Design review of the part built by this model. Coordinates are the model's own, in mm. Face numbers are marked on the shaded views. A direction names the side the tool comes from. Round coordinates to 2 decimals unless told otherwise and drop trailing zeros. Write each loop counter-clockwise with the first axis right and the second up, starting at its lowest first coordinate (ties: lowest second). Pieces come first, ordered by that corner, then holes. Notation, with made-up numbers: M 6.5,-25.5 L 12.5,-25.5 A34 ccw 12.5,4.5 Z; hole C 61.25,44 d9. An arc over 180 degrees is marked long. One line per question, with ' | ' between items. Start each with the question number.
Item 1: Add section B-B, the plane y = 10. State the section outline as (x, z) points.
Item 2: Insertion check: pin 1 Ø5 at (x, z) = (3, -9) entering from -Y; pin 2 Ø5 at (x, y) = (18, 0) entering from +Z; pin 3 Ø5 at (x, y) = (-26.5, 4) entering from +Z; pin 4 Ø1 at (x, y) = (-5, 11) entering from +Z. Each pin has a flat end and moves straight along its axis. Give the tip position at first contact, or say it passes through.
Item 3: For L1, parallel to Y at x = 0, z = -10; L2, parallel to Y at x = -18, z = -39.25; L3, parallel to Y at x = 30, z = -30, list the stretches that pass through material, from the lowest coordinate up.
Item 4: Add section C-C, the plane x = -18. Give the number of separate pieces and of enclosed holes in the cut face, and give its area (3 significant figures).
Item 5: Add section A-A, the plane x = 0. State the section outline as (y, z) points.
Item 6: Draft analysis for pull direction Y (two halves, no side actions). For the marked faces 4, 5 and 6, state which applies: released by +Y, released by -Y, zero draft, split by the parting line, or undercut.
Item 7: Machinability: for the marked faces 1, 2 and 3, which of the approach directions +Z, -Z, +X, -X, +Y, -Y give a long, thin tool a straight path to every point of the face, cutting with its end or side? Answer none if there is none.
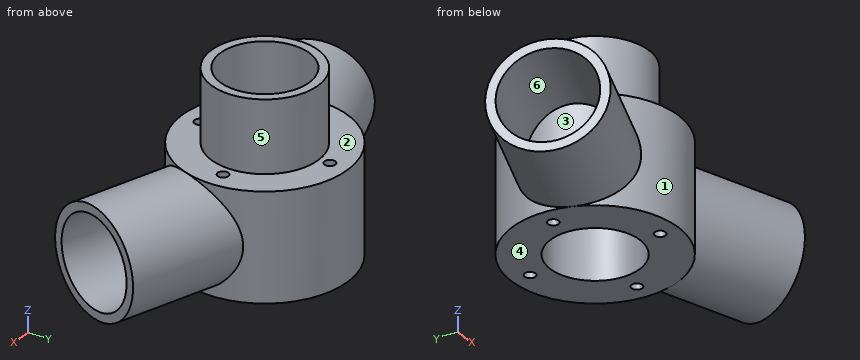
```python
from build123d import *

# Parameters (mm, degrees)
CROQUIS1_R              = 15
CROQUIS1_R_2            = 12.5
SALIENTE_EXTRUIR1_DEPTH = 20
CROQUIS8_R              = 23.25
CROQUIS8_R_2            = 1.5
SALIENTE_EXTRUIR2_DEPTH = 30
SALIENTE_EXTRUIR4_REACH = 81.8
CROQUIS6_R              = 15
CROQUIS6_R_2            = 12.5
SALIENTE_EXTRUIR5_REACH = 108.924
CROQUIS7_R              = 15
CROQUIS7_R_2            = 12.5
CROQUIS9_R              = 12.5
CORTAR_EXTRUIR1_DEPTH   = 31.000000103


with BuildPart() as part:
    # Croquis1 → Saliente-Extruir1 (new body)
    with BuildSketch(Plane.XY):
        Circle(CROQUIS1_R)
        Circle(CROQUIS1_R_2, mode=Mode.SUBTRACT)
    extrude(amount=-SALIENTE_EXTRUIR1_DEPTH)

    # Croquis8 → Saliente-Extruir2 (add)
    with BuildSketch(Plane(origin=(0, 0, -20), x_dir=(-1, 0, 0), z_dir=(0, 0, -1))):
        Circle(CROQUIS8_R)
        with Locations((0, 18)):
            Circle(CROQUIS8_R_2, mode=Mode.SUBTRACT)
        with Locations((18, 0)):
            Circle(CROQUIS8_R_2, mode=Mode.SUBTRACT)
        with Locations((0, -18)):
            Circle(CROQUIS8_R_2, mode=Mode.SUBTRACT)
        with Locations((-18, 0)):
            Circle(CROQUIS8_R_2, mode=Mode.SUBTRACT)
    extrude(amount=SALIENTE_EXTRUIR2_DEPTH)

    # Croquis6 → Saliente-Extruir4 (add, up to next)
    with BuildSketch(Plane(origin=(46.984631039, -17.101007166, -35), x_dir=(0, 0, -1), z_dir=(0.939692621, -0.342020143, 0)), mode=Mode.PRIVATE) as saliente_extruir4_sk1:
        Circle(CROQUIS6_R)
        Circle(CROQUIS6_R_2, mode=Mode.SUBTRACT)
    saliente_extruir4_tool1 = extrude(saliente_extruir4_sk1.sketch, amount=-SALIENTE_EXTRUIR4_REACH, mode=Mode.PRIVATE) - part.part
    add(saliente_extruir4_tool1.solids().sort_by_distance((46.984631, -17.101007, -20.424264))[0])

    # Croquis7 → Saliente-Extruir5 (add, up to next)
    with BuildSketch(Plane(origin=(-46.984631039, -17.101007166, -35), x_dir=(0, 0, 1), z_dir=(-0.939692621, -0.342020143, 0)), mode=Mode.PRIVATE) as saliente_extruir5_sk1:
        Circle(CROQUIS7_R)
        Circle(CROQUIS7_R_2, mode=Mode.SUBTRACT)
    saliente_extruir5_tool1 = extrude(saliente_extruir5_sk1.sketch, amount=-SALIENTE_EXTRUIR5_REACH, mode=Mode.PRIVATE) - part.part
    add(saliente_extruir5_tool1.solids().sort_by_distance((-46.984631, -17.101007, -49.575736))[0])

    # Croquis9 → Cortar-Extruir1 (cut, through all)
    with BuildSketch(Plane.XY.offset(-20)):
        Circle(CROQUIS9_R)
    extrude(amount=-CORTAR_EXTRUIR1_DEPTH, mode=Mode.SUBTRACT)


solid = part.part
```
Computed values:
1) outline: M -20.99,-50 L -7.5,-50 L -7.5,0 L -11.18,0 L -11.18,-20 L -20.99,-20 Z; M 7.5,-50 L 20.99,-50 L 20.99,-20 L 11.18,-20 L 11.18,0 L 7.5,0 Z
2) pin 1: stops at y = -14.99 | pin 2: stops at z = -20 | pin 3: stops at z = -24.12 | pin 4: stops at z = 0
3) L1: y = -15 to -12.5, 12.5 to 15 | L2: y = -21.86 to -19.06, -14.72 to -1.5, 1.5 to 14.72 | L3: y = -25.97 to -23.11, 1.27 to 4.13
4) separate pieces: 2 | enclosed holes: 1 | area: 865 mm^2
5) outline: M -23.25,-50 L -19.5,-50 L -19.5,-20 L -23.25,-20 Z; M -16.5,-50 L -12.5,-50 L -12.5,0 L -15,0 L -15,-20 L -16.5,-20 Z; M 12.5,-50 L 16.5,-50 L 16.5,-20 L 15,-20 L 15,0 L 12.5,0 Z; M 19.5,-50 L 23.25,-50 L 23.25,-20 L 19.5,-20 Z
6) face 4: zero draft | face 5: split by the parting line | face 6: undercut
7) face 1: -Y | face 2: +Z | face 3: none
